```python
from build123d import *

# Parameters (mm, degrees)
F1_DEPTH = 160
F3_T     = -1.8
F4_DEPTH = 1.8


with BuildPart() as f1:
    # F0 (on Front) → F1 (new body)
    with BuildSketch(Plane.XZ):
        Polygon((-40, 0), (-40, -40), (-10, -40), (10, -40), (40, -40), (40, 15), (-40, 15), align=None)
    extrude(amount=F1_DEPTH)

    # F3
    f3_openings = [f1.faces().sort_by_distance(p)[0] for p in [
        (0, -80, 15),
        (0, -80, -40),
    ]]
    offset(amount=F3_T, openings=f3_openings)

    # F2 (on Front) → F4 (cut)
    with BuildSketch(Plane.XZ):
        Polygon((10, -5), (0, -5), (-10, -5), (-10, -40), (10, -40), align=None)
    extrude(amount=F4_DEPTH, mode=Mode.SUBTRACT)


solid = f1.part
```
The listing builds one solid part. Answer for the finished solid, in the listing's coordinates (mm). A direction names the side the tool comes from. Give positions to 0.01 mm unless a question says otherwise; leave off trailing zeros. Order: outer loops, then holes, each group sorted by start corner. A loop starts at its lowest first (then second) coordinate and runs counter-clockwise, first axis right, second up. Notation, with made-up numbers: (25, 69.25) - (37, 69.25) arc R24 ccw to (37, 85.25) - close; hole circle Ø3 at (-0.5, 20). An arc over 180 degrees is marked (long way). Use one line per item in the form item = value. Start each with the question number.
(1) A cutting plane is placed at C-C, the plane z = 2. Write down the section's boundary in (x, y), then the cut area to 3 significant figures.
(2) Consider line 1 (X direction, y = -81, z = 11.5); line 2 (Y direction, x = 7, z = 5); line 3 (Y direction, x = -8, z = -21). Determine where each line is inside the solid, lowest interval first. Write a range as from..to.
(3) The mould has two halves that part along Y. Classify faces 3 (the flat face through (-1, -158.2, -12)), 4 (the flat face through (-1, -1.8, 0)), 5 (the flat face through (40, -79, -13)), 6 (the flat face through (-1, 0, 0)): released by +Y, released by -Y, zero draft, split by the parting line, or undercut.
(4) A cutting plane is placed at D-D, the plane z = -17. Write down the section's boundary in (x, y).
(5) A flat-ended cylindrical pin translates along its axis: pin 1 Ø1.4 at (x, y) = (5, -0.5) entering from -Z. Find the tip coordinate at first contact, or state that the pin passes through.
(6) A cutting plane is placed at B-B, the plane x = -2. Write down the section's boundary in (y, z).
(7) For faces 1 (the flat face through (-40, -79, -12)), 2 (the flat face through (-38.2, -79, -12)), determine the directions among +Z, -Z, +X, -X, +Y, -Y from which every point of the face is accessible in a straight line to the end or side of a thin tool.
(8) A cutting plane is placed at A-A, the plane y = -15. Write down the section's boundary in (x, z), then the cut area to 3 significant figures.
Ans:
q1.outline = (-40, -160) - (40, -160) - (40, 0) - (-40, 0) - close; hole (-38.2, -158.2) - (38.2, -158.2) - (38.2, -1.8) - (-38.2, -1.8) - close
q1.area = 851 mm^2
q2.line_1 = -40..-38.2, 38.2..40
q2.line_2 = -160..-158.2, -1.8..0
q2.line_3 = -160..-158.2
q3.face_3 = undercut
q3.face_4 = undercut
q3.face_5 = zero draft
q3.face_6 = released by +Y
q4.outline = (-40, -160) - (40, -160) - (40, 0) - (10, 0) - (10, -1.8) - (38.2, -1.8) - (38.2, -158.2) - (-38.2, -158.2) - (-38.2, -1.8) - (-10, -1.8) - (-10, 0) - (-40, 0) - close
q5.pin_1 = -5
q6.outline = (-160, -40) - (-158.2, -40) - (-158.2, 15) - (-160, 15) - close; (-1.8, -5) - (0, -5) - (0, 15) - (-1.8, 15) - close
q7.face_1 = +Z, -Z, -X, +Y, -Y
q7.face_2 = +Z, -Z
q8.outline = (-40, -40) - (-38.2, -40) - (-38.2, 15) - (-40, 15) - close; (38.2, -40) - (40, -40) - (40, 15) - (38.2, 15) - close
q8.area = 198 mm^2
